Input: part model. Units: mm. Frame: model coordinates. Face numbers are marked on the shaded views. A direction names the side the tool comes from. Give positions to 0.01 mm unless a question says otherwise; leave off trailing zeros. Loops run counter-clockwise (first coordinate to the right, second up) from the corner with the lowest first, then second, coordinate; pieces in that order, holes last. Notation, with made-up numbers: (-22.5, -30.75) -> (36.5, -30.75) arc R12 ccw to (36.5, -8.75) -> close; hole circle Ø8 at (53, -16.5). An arc over 180 degrees is marked (long way). Answer as a JSON object with one key per item and string values.
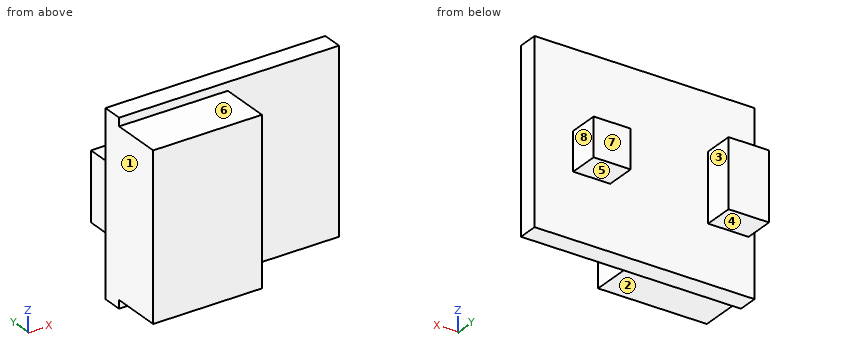
```python
from build123d import *

# Parameters (mm, degrees)
F0_W     = 10.874254629
F0_H     = 16.3510471284
F1_DEPTH = 2
F2_DEPTH = 7
F3_W     = 4.0485225618
F3_H     = 6.7925304174
F3_W_2   = 3.7012062967
F3_H_2   = 3.8396660239
F4_DEPTH = 3


with BuildPart() as f1:
    # F0 (on Front) → F1 (new body)
    with BuildSketch(Plane.XZ):
        Polygon((-19.8561436236, -13.0616642237), (-41.8561436236, -13.0616642237), (-41.8561436236, -13.8861406595), (-30.9818889946, -13.8861406595), (-30.9818889946, -30.2371877879), (-41.8561436236, -30.2371877879), (-41.8561436236, -31.0616642237), (-19.8561436236, -31.0616642237), align=None)
        with Locations((-36.4190163091, -22.0616642237)):
            Rectangle(F0_W, F0_H)
    extrude(amount=F1_DEPTH)

    # F0 (on Front) → F2 (join)
    with BuildSketch(Plane.XZ):
        with Locations((-36.4190163091, -22.0616642237)):
            Rectangle(F0_W, F0_H)
    extrude(amount=F2_DEPTH)

    # F3 (on face) → F4 (join)
    with BuildSketch(Plane(origin=(0, 0, 0), x_dir=(-1, 0, 0), z_dir=(0, 1, 0))):
        with Locations((39.2332170159, -21.982813254)):
            Rectangle(F3_W, F3_H)
        with Locations((25.5681611598, -22.7285558358)):
            Rectangle(F3_W_2, F3_H_2)
    extrude(amount=F4_DEPTH)


solid = f1.part
```
Q1. Section A-A, the plane y = 0.25. Return the cut outline in (x, z), then the cut area to 3 significant figures.
Evaluation:
{"outline": "(-41.26, -25.38) -> (-37.21, -25.38) -> (-37.21, -18.59) -> (-41.26, -18.59) -> close; (-27.42, -24.65) -> (-23.72, -24.65) -> (-23.72, -20.81) -> (-27.42, -20.81) -> close", "area": "41.7 mm2"}
Q2. Section D-D, the plane y = -5. Return the cut outline in (x, z).
Evaluation:
{"outline": "(-41.86, -30.24) -> (-30.98, -30.24) -> (-30.98, -13.89) -> (-41.86, -13.89) -> close"}
Q3. Access query for the marked faces 4, 5, 6, 7 and 8. Directions: +Z, -Z, +X, -X, +Y, -Y. A direction counts if a zero-diameter tool reaches every point of the face in a straight line with its end or side. Return the directions, or none.
Evaluation:
{"face 4": "-Z, +X, -X, +Y", "face 5": "-Z, +X, +Y", "face 6": "+Z, +X, -X, -Y", "face 7": "+Z, -Z, +X, -X, +Y", "face 8": "+Z, -Z, +X, +Y"}
Q4. Section C-C, the plane z = -22.25. Return the cut outline in (x, y).
Evaluation:
{"outline": "(-41.86, -7) -> (-30.98, -7) -> (-30.98, -2) -> (-19.86, -2) -> (-19.86, 0) -> (-23.72, 0) -> (-23.72, 3) -> (-27.42, 3) -> (-27.42, 0) -> (-37.21, 0) -> (-37.21, 3) -> (-41.26, 3) -> (-41.26, 0) -> (-41.86, 0) -> close"}
Q5. Draft query along X for the marked faces 1, 2 and 3. Return one class per face: +X half, -X half, draft (parallel to the pull), parting line (faces both ways), or undercut.
Evaluation:
{"face 1": "-X half", "face 2": "draft", "face 3": "undercut"}
Q6. Ray query, line 1 along X through (y, z) = (-6, -25.5); line 2 along Y through (x, z) = (-29, -26.75); line 3 along Y through (x, z) = (-31.25, -17.25). Return the intervals inside material, ascending.
Evaluation:
{"line 1": "x = -41.86 to -30.98", "line 2": "y = -2 to 0", "line 3": "y = -7 to 0"}
Q7. Section B-B, the plane x = -32. Return the cut outline in (y, z).
Evaluation:
{"outline": "(-7, -30.24) -> (-2, -30.24) -> (-2, -31.06) -> (0, -31.06) -> (0, -13.06) -> (-2, -13.06) -> (-2, -13.89) -> (-7, -13.89) -> close"}
Q8. Pin query (flat end, axial travel): pin 1 (3.5 mm diameter, centred on y = 2, z = -21, fed in from -X); pin 2 (0.9 mm diameter, centred on y = 1, z = -23, fed in from +X); pin 3 (0.9 mm diameter, centred on x = -39, y = 1.5, fed in from +Z). Return the tip coordinate at first contact, or that it passes through.
Evaluation:
{"pin 1": "stops at x = -41.26", "pin 2": "stops at x = -23.72", "pin 3": "stops at z = -18.59"}
